The listing builds one solid part. Answer for the finished solid, in the listing's coordinates (mm). Face numbers are marked on the shaded views. A direction names the side the tool comes from. Round coordinates to 2 decimals unless told otherwise and drop trailing zeros. Order: outer loops, then holes, each group sorted by start corner. A loop starts at its lowest first (then second) coordinate and runs counter-clockwise, first axis right, second up. Notation, with made-up numbers: (-33.5, 72.5) -> (-26.5, 72.5) arc R31 ccw to (-26.5, 101.5) -> close; hole circle Ø2 at (71.5, 7.5). An arc over 180 degrees is marked (long way). Return JSON: item names as keys, results as strings. Group by question number.
(1) The part is cut by section A-A (z = 56.5). Determine the outline of the cut face in (x, y).
(2) Determine the mould class of the marked faces 3, 4 and 5 for opening direction Y: +Y half, -Y half, draft (parallel to the pull), parting line (faces both ways), or undercut.
(3) The part is cut by section C-C (z = 102). Determine the outline of the cut face in (x, y), plus the area to 3 significant figures.
(4) Which of the six approach directions +Z, -Z, +X, -X, +Y, -Y give full straight-line access (tool end or side, diameter ignored) to the marked faces 1 and 2?
(5) The part is cut by section B-B (x = 86). Determine the outline of the cut face in (y, z).
(6) Consider line 1 (X direction, y = 224.5, z = 176); line 2 (Y direction, x = -82.5, z = 110). Determine where each line is inside the solid, lowest interval first. Write a range as [from, to].
(7) Each of these flat-tipped pins is pushed along its axis until it touches: pin 1 (0.8 mm diameter, centred on y = 280.5, z = 179.5, fed in from +X); pin 2 (3 mm diameter, centred on x = 16.5, y = 44.5, fed in from +Z); pin 3 (6.5 mm diameter, centred on x = -134, z = 166, fed in from +Y). Where does it stop, or does it pass through?
(8) The part is cut by section D-D (y = -165). Determine the outline of the cut face in (x, z).
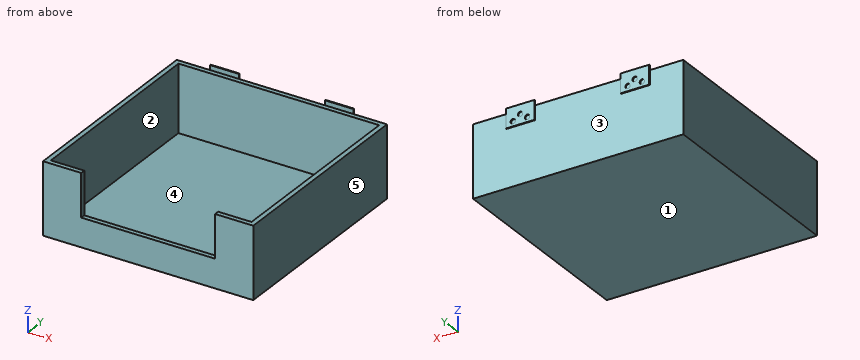
from build123d import *

# Parameters (mm, degrees)
F0_W      = 558.8
F0_H      = 558.8
F1_DEPTH  = 12.7
F2_W      = 12.7
F2_H      = 546.1
F3_DEPTH  = 177.8
F4_W      = 533.4
F4_H      = 12.7
F5_DEPTH  = 63.5
F6_W      = 88.9
F6_H      = 12.7
F7_DEPTH  = 114.3
F8_W      = 76.2
F8_H      = 38.1
F9_DEPTH  = 2.54
F10_W     = 76.2
F10_H     = 2.54
F11_DEPTH = 12.7
F13_DEPTH = 2.54
F15_DEPTH = 2.54


with BuildPart() as f1:
    # F0 (on Top) → F1 (new body)
    with BuildSketch(Plane.XY):
        Rectangle(F0_W, F0_H)
    extrude(amount=F1_DEPTH)

    # F2 (on face) → F3 (join)
    with BuildSketch(Plane.XY.offset(12.7)):
        with Locations((-273.05, -6.35)):
            Rectangle(F2_W, F2_H)
        Polygon((279.4, 279.4), (-279.4, 279.4), (-279.4, 266.7), (-266.7, 266.7), (266.7, 266.7), (279.4, 266.7), align=None)
        with Locations((273.05, -6.35)):
            Rectangle(F2_W, F2_H)
    extrude(amount=F3_DEPTH)

    # F4 (on face) → F5 (join)
    with BuildSketch(Plane.XY.offset(12.7)):
        with Locations((0, -273.05)):
            Rectangle(F4_W, F4_H)
    extrude(amount=F5_DEPTH)

    # F6 (on face) → F7 (join)
    with BuildSketch(Plane.XY.offset(76.2)):
        with Locations((-222.25, -273.05)):
            Rectangle(F6_W, F6_H)
        with Locations((222.25, -273.05)):
            Rectangle(F6_W, F6_H)
    extrude(amount=F7_DEPTH)

    # F8 (on face) → F9 (join)
    with BuildSketch(Plane(origin=(0, 279.4, 0), x_dir=(-1, 0, 0), z_dir=(0, 1, 0))):
        with Locations((-152.4, 171.45)):
            Rectangle(F8_W, F8_H)
        with Locations((152.4, 171.45)):
            Rectangle(F8_W, F8_H)
    extrude(amount=F9_DEPTH)

    # F10 (on face) → F11 (join)
    with BuildSketch(Plane.XY.offset(190.5)):
        with Locations((-152.4, 280.67)):
            Rectangle(F10_W, F10_H)
        with Locations((152.4, 280.67)):
            Rectangle(F10_W, F10_H)
    extrude(amount=F11_DEPTH)

    # F12 (on face) → F13 (cut)
    with BuildSketch(Plane(origin=(0, 281.94, 0), x_dir=(-1, 0, 0), z_dir=(0, 1, 0))):
        with BuildLine():
            Line((-171.45, 158.75), (-171.45, 171.45))
            ThreePointArc((-171.45, 171.45), (-177.8, 165.1), (-171.45, 158.75))
        make_face()
        with BuildLine():
            ThreePointArc((-165.1, 165.1), (-166.9598719395, 169.5901280605), (-171.45, 171.45))
            Line((-171.45, 171.45), (-171.45, 158.75))
            ThreePointArc((-171.45, 158.75), (-166.9598719395, 160.6098719395), (-165.1, 165.1))
        make_face()
        with BuildLine():
            ThreePointArc((-152.4, 184.15), (-156.8901280605, 182.2901280605), (-158.75, 177.8))
            Line((-158.75, 177.8), (-152.4, 177.8))
            Line((-152.4, 177.8), (-152.4, 184.15))
        make_face()
        with BuildLine():
            Line((-152.4, 177.8), (-158.75, 177.8))
            ThreePointArc((-158.75, 177.8), (-156.8901280605, 173.3098719395), (-152.4, 171.45))
            Line((-152.4, 171.45), (-152.4, 177.8))
        make_face()
        with BuildLine():
            Line((-146.05, 177.8), (-152.4, 177.8))
            Line((-152.4, 177.8), (-152.4, 171.45))
            ThreePointArc((-152.4, 171.45), (-147.9098719395, 173.3098719395), (-146.05, 177.8))
        make_face()
        with BuildLine():
            Line((-152.4, 184.15), (-152.4, 177.8))
            Line((-152.4, 177.8), (-146.05, 177.8))
            ThreePointArc((-146.05, 177.8), (-147.9098719395, 182.2901280605), (-152.4, 184.15))
        make_face()
        with BuildLine():
            ThreePointArc((-133.35, 171.45), (-139.7, 165.1), (-133.35, 158.75))
            Line((-133.35, 158.75), (-133.35, 171.45))
        make_face()
        with BuildLine():
            Line((-133.35, 171.45), (-133.35, 158.75))
            ThreePointArc((-133.35, 158.75), (-128.8598719395, 160.6098719395), (-127, 165.1))
            ThreePointArc((-127, 165.1), (-128.8598719395, 169.5901280605), (-133.35, 171.45))
        make_face()
    extrude(amount=-F13_DEPTH, mode=Mode.SUBTRACT)

    # F14 (on face) → F15 (cut)
    with BuildSketch(Plane(origin=(0, 281.94, 0), x_dir=(-1, 0, 0), z_dir=(0, 1, 0))):
        with BuildLine():
            Line((152.4, 184.15), (152.4, 177.8))
            Line((152.4, 177.8), (158.75, 177.8))
            ThreePointArc((158.75, 177.8), (156.8901280605, 182.2901280605), (152.4, 184.15))
        make_face()
        with BuildLine():
            ThreePointArc((152.4, 184.15), (147.9098719395, 182.2901280605), (146.05, 177.8))
            Line((146.05, 177.8), (152.4, 177.8))
            Line((152.4, 177.8), (152.4, 184.15))
        make_face()
        with BuildLine():
            Line((152.4, 177.8), (146.05, 177.8))
            ThreePointArc((146.05, 177.8), (147.9098719395, 173.3098719395), (152.4, 171.45))
            Line((152.4, 171.45), (152.4, 177.8))
        make_face()
        with BuildLine():
            Line((158.75, 177.8), (152.4, 177.8))
            Line((152.4, 177.8), (152.4, 171.45))
            ThreePointArc((152.4, 171.45), (156.8901280605, 173.3098719395), (158.75, 177.8))
        make_face()
        with BuildLine():
            ThreePointArc((139.7, 165.1), (137.8401280605, 169.5901280605), (133.35, 171.45))
            Line((133.35, 171.45), (133.35, 158.75))
            ThreePointArc((133.35, 158.75), (137.8401280605, 160.6098719395), (139.7, 165.1))
        make_face()
        with BuildLine():
            Line((133.35, 158.75), (133.35, 171.45))
            ThreePointArc((133.35, 171.45), (127, 165.1), (133.35, 158.75))
        make_face()
        with BuildLine():
            ThreePointArc((171.45, 171.45), (165.1, 165.1), (171.45, 158.75))
            Line((171.45, 158.75), (171.45, 171.45))
        make_face()
        with BuildLine():
            Line((171.45, 171.45), (171.45, 158.75))
            ThreePointArc((171.45, 158.75), (175.9401280605, 160.6098719395), (177.8, 165.1))
            ThreePointArc((177.8, 165.1), (175.9401280605, 169.5901280605), (171.45, 171.45))
        make_face()
    extrude(amount=-F15_DEPTH, mode=Mode.SUBTRACT)


solid = f1.part
Answer below:
{
 "1": {"outline": "(-279.4, -279.4) -> (279.4, -279.4) -> (279.4, 279.4) -> (-279.4, 279.4) -> close; hole (-266.7, -266.7) -> (266.7, -266.7) -> (266.7, 266.7) -> (-266.7, 266.7) -> close"},
 "2": {"face 3": "+Y half", "face 4": "undercut", "face 5": "draft"},
 "3": {"outline": "(-279.4, -279.4) -> (-177.8, -279.4) -> (-177.8, -266.7) -> (-266.7, -266.7) -> (-266.7, 266.7) -> (266.7, 266.7) -> (266.7, -266.7) -> (177.8, -266.7) -> (177.8, -279.4) -> (279.4, -279.4) -> (279.4, 279.4) -> (-279.4, 279.4) -> close", "area": "23,200 mm²"},
 "4": {"face 1": "-Z, +X, -X, +Y, -Y", "face 2": "+Z"},
 "5": {"outline": "(-279.4, 0) -> (279.4, 0) -> (279.4, 190.5) -> (266.7, 190.5) -> (266.7, 12.7) -> (-266.7, 12.7) -> (-266.7, 76.2) -> (-279.4, 76.2) -> close"},
 "6": {"line 1": "x = [-279.4, -266.7], [266.7, 279.4]", "line 2": "y = [266.7, 279.4]"},
 "7": {"pin 1": "stops at x = 190.5", "pin 2": "stops at z = 12.7", "pin 3": "stops at y = 279.4"},
 "8": {"outline": "(-279.4, 0) -> (279.4, 0) -> (279.4, 190.5) -> (266.7, 190.5) -> (266.7, 12.7) -> (-266.7, 12.7) -> (-266.7, 190.5) -> (-279.4, 190.5) -> close"}
}
